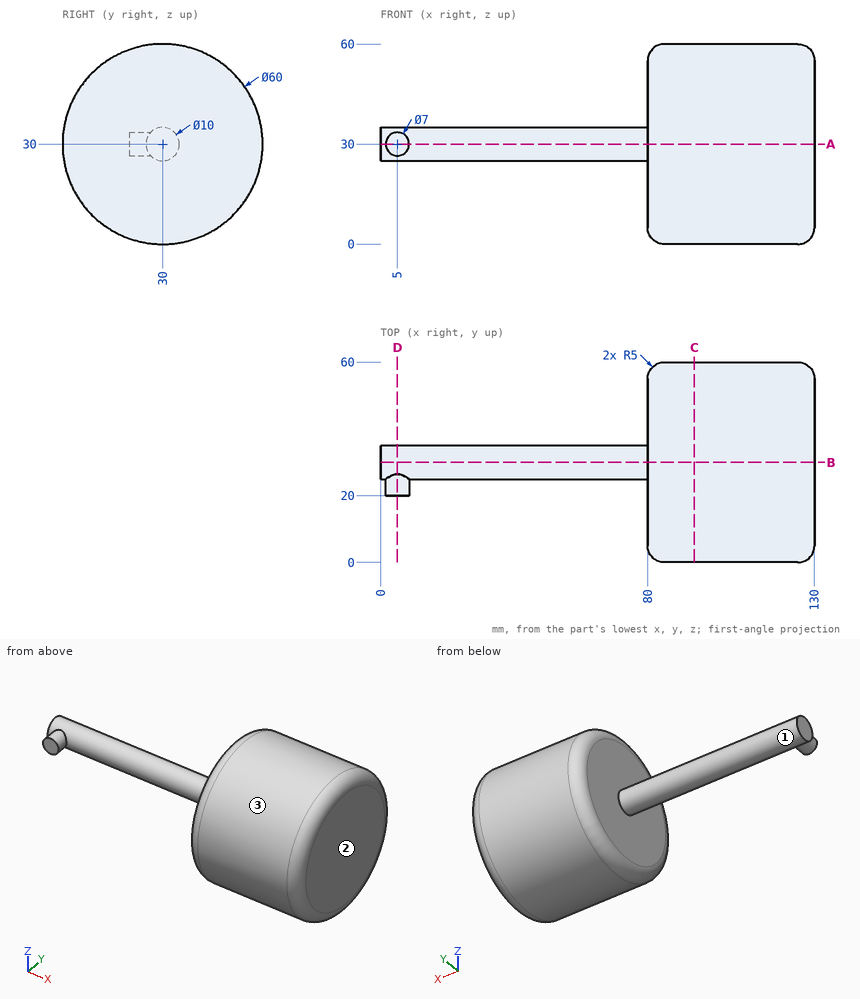
Input: dimensioned drawing with shaded views. Units: mm. Origin: part minimum x, y, z. Round coordinates to 2 decimals unless told otherwise and drop trailing zeros. Order: outer loops, then holes, each group sorted by start corner. A loop starts at its lowest first (then second) coordinate and runs counter-clockwise, first axis right, second up. Notation, with made-up numbers: (-39, 25.5) -> (9, 25.5) arc R31 cw to (9, 55.5) -> close; hole circle Ø7 at (-21.5, 0). An arc over 180 degrees is marked (long way). Put each result on its own line as item: value. Start each with the question number.
Q1. Section C-C on x = 94. Return the cut outline in (y, z).
Q2. Section A-A on z = 30. Return the cut outline in (x, y).
Q3. Section B-B on y = 30. Return the cut outline in (x, z).
Q4. Line query: probe 1 along X at (y, z) = (43, 11.5); probe 2 along Y at (x, z) = (111, 4); probe 3 along Z at (x, y) = (35.5, 28.5). Output: solid intervals per line, ascending.
Q5. First-contact query: pin 1 (1.5 mm diameter, centred on x = 103.5, y = 41, fed in from +Z); pin 2 (2 mm diameter, centred on x = 6.5, z = 31.5, fed in from -Y); pin 3 (10 mm diameter, centred on x = 102, y = 9, fed in from +Z). Flat tips, straight axial feed; report the tip coordinate or a pass-through.
Q6. Section D-D on x = 5. Return the cut outline in (y, z), and give its area (3 significant figures).
Q7. Pull-direction query (X, two-part tool) for the marked faces 1, 2 and 3; classes: +X half, -X half, draft (parallel to the pull), parting line (faces both ways), or undercut.
Ans:
1. outline: circle Ø60 at (30, 30)
2. outline: (0, 25) -> (1.5, 25) -> (1.5, 20) -> (8.5, 20) -> (8.5, 25) -> (80, 25) -> (80, 5) arc R5 ccw to (85, 0) -> (125, 0) arc R5 ccw to (130, 5) -> (130, 55) arc R5 ccw to (125, 60) -> (85, 60) arc R5 ccw to (80, 55) -> (80, 35) -> (0, 35) -> close
3. outline: (0, 25) -> (80, 25) -> (80, 5) arc R5 ccw to (85, 0) -> (125, 0) arc R5 ccw to (130, 5) -> (130, 55) arc R5 ccw to (125, 60) -> (85, 60) arc R5 ccw to (80, 55) -> (80, 35) -> (0, 35) -> close
4. probe 1: x = 80 to 130
4. probe 2: y = 15.03 to 44.97
4. probe 3: z = 25.23 to 34.77
5. pin 1: stops at z = 58.19
5. pin 2: stops at y = 20
5. pin 3: stops at z = 55.38
6. outline: (20, 26.5) -> (26.43, 26.5) arc R5 ccw (long way) to (26.43, 33.5) -> (20, 33.5) -> close
6. area: 117 mm2
7. face 1: undercut
7. face 2: +X half
7. face 3: draft
